from build123d import *

# Parameters (mm, degrees)
F0_R            = 50.8
F1_DEPTH        = 12.7
F3_DEPTH        = 25.4
F3_COPIES_COUNT = 30


# Not quite as in the source:
# - a pattern or mirror of a feature is missing from the dataset's text; its kind, count and spacing are read off the source's solid


with BuildPart() as f1:
    # F0 (on Front) → F1 (new body, symmetric)
    with BuildSketch(Plane.XZ):
        Circle(F0_R)
    extrude(amount=F1_DEPTH, both=True)

    # F2 (on face) → F3 (join)
    with BuildSketch(Plane.XZ.offset(12.7)):
        with BuildLine():
            ThreePointArc((0, 50.8), (5.310045934, 50.5217122847), (10.5619138935, 49.6898981173))
            Line((10.5619138935, 49.6898981173), (6.1639756896, 59.2651665211))
            Line((6.1639756896, 59.2651665211), (0, 50.8))
        make_face()
    f3 = extrude(amount=-F3_DEPTH)

    # F3_copies: F3 ×30 about axis
    f3_copies_axis = Axis((0, 0, 0), (0, 1, 0))
    for i in range(1, F3_COPIES_COUNT):
        add(f3.rotate(f3_copies_axis, i * 360 / F3_COPIES_COUNT))


solid = f1.part
Could you check a few things on this model? Use its own coordinates, in mm. A direction names the side the tool comes from. Give positions to 0.01 mm unless a question says otherwise; leave off trailing zeros. Order: outer loops, then holes, each group sorted by start corner. A loop starts at its lowest first (then second) coordinate and runs counter-clockwise, first axis right, second up. Notation, with made-up numbers: (48.5, -33.75) -> (106.5, -33.75) arc R7 cw to (106.5, -24.75) -> close; hole circle Ø8 at (14.25, 43.25). An arc over 180 degrees is marked (long way). Return JSON: item names as keys, results as strings.
1. Imagine slicing it at B-B on x = -9. List the corners of the cut face in (y, z) for me, then the cut area to 3 significant figures.
Answer list:
{"outline": "(-12.7, -53.09) -> (12.7, -53.09) -> (12.7, 53.19) -> (-12.7, 53.19) -> close", "area": "2,700 mm2"}
2. Thinking about a two-plate mould opening in Z: for faces 1 (the flat face through (-55.12, -0.18, -2.65)), 2 (the flat face through (14.511, -0.178, 53.238)), 3 (the flat face through (3.102, -0.178, -54.967)), which applies, pulls with the +Z half, pulls with the -Z half, needs draft (parallel to the pull), parting line crosses it, or undercut?
Answer list:
{"face 1": "undercut", "face 2": "pulls with the +Z half", "face 3": "pulls with the -Z half"}
3. I need wall thicknesses on line 1 (Z direction, x = 53, y = -2.5); line 2 (Z direction, x = 45.5, y = -1.25); line 3 (Z direction, x = 47, y = 6.5). Which ranges of each line are inside material? Lowest first, please. Write a range as from..to.
Answer list:
{"line 1": "z = -24.35..-22.16, -14.11..-7.55, -3.84..3.88, 7.59..14.17, 22.31..24.44", "line 2": "z = -34.71..-28.79, -25.22..25.24, 28.89..34.8", "line 3": "z = -34.85..-32.17, -25.05..25.08, 32.37..34.95"}
4. Imagine slicing it at A-A on z = -20.5. List the corners of the cut face in (x, y) for me.
Answer list:
{"outline": "(-51.72, -12.7) -> (51.79, -12.7) -> (51.79, 12.7) -> (-51.72, 12.7) -> close"}
5. On a 3-axis mill with a long thin cutter (end or side, diameter ignored), from which of +Z, -Z, +X, -X, +Y, -Y can I reach the whole of each face in a straight line? I mean faces 4 (the flat face through (-49.27, -0.18, -24.84)), 5 (the flat face through (51.32, -0.18, 19.94)), 6 (the flat face through (-34.91, -0.178, -42.733)). Say none if no direction works.
Answer list:
{"face 4": "-X, +Y, -Y", "face 5": "+X, +Y, -Y", "face 6": "-Z, +Y, -Y"}
6. For pin 1 Ø2 at (y, z) = (8.5, -9.5) entering from +X; pin 2 Ø5 at (y, z) = (2, 25.5) entering from +X; pin 3 Ø5 at (y, z) = (8.5, -39.5) entering from -X, each with a flat end and sliding along its axis, tell me the tip position at first contact or that it passes through.
Answer list:
{"pin 1": "stops at x = 56.27", "pin 2": "stops at x = 54.41", "pin 3": "stops at x = -39.36"}
